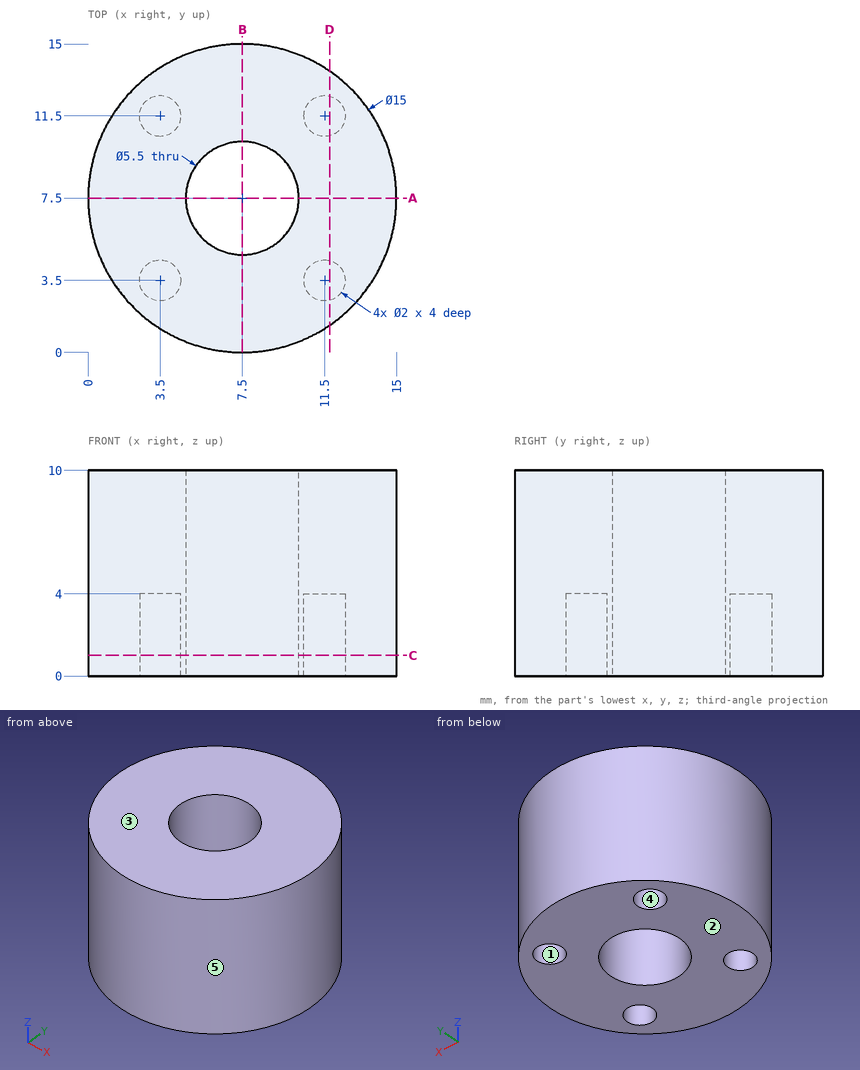
Study the drawing (mm; zero at the part's minimum x, y, z) and answer. A direction names the side the tool comes from. Round coordinates to 2 decimals unless told otherwise and drop trailing zeros. Write each loop counter-clockwise with the first axis right and the second up, starting at its lowest first coordinate (ties: lowest second). Pieces come first, ordered by that corner, then holes. Notation, with made-up numbers: (-2, 77) - (20, 77) arc R24 cw to (20, 113) - close; hole circle Ø9 at (-8.5, 39). An arc over 180 degrees is marked (long way). Use a Markdown table: item, result. Add a question column.
1. Flat-ended cylindrical pins translate along their axes: P1, Ø5, axis at x = 13, z = 4, coming from the +Y side; P2, Ø2, axis at x = 11.5, y = 11, coming from the -Z side; P3, Ø1.5, axis at x = 6, z = 3.5, coming from the -Y side; P4, Ø1.5, axis at y = 11, z = 2.5, coming from the -X side. Find the tip coordinate at first contact, or state that the pin passes through.
2. Consider line 1 (X direction, y = 4, z = 0.5); line 2 (Y direction, x = 3.5, z = 2.75); line 3 (Y direction, x = 7.5, z = 2.5). Determine where each line is inside the solid, lowest interval first.
3. The part is cut by section C-C (z = 1). Write down the section's boundary in (x, y).
4. For a pull along X with two mould halves and no side action, classify the marked faces 3, 4 and 5 as +X half, -X half, draft (parallel to the pull), parting line (faces both ways), or undercut.
5. A tool of negligible diameter and unlimited length cuts with its end or side. For the marked faces 1 and 2, from which of +Z, -Z, +X, -X, +Y, -Y can it reach the whole face along a straight path? Write none if from no direction.
6. The part is cut by section D-D (x = 11.75). Write down the section's boundary in (y, z), and give its area (3 significant figures).
7. The part is cut by section A-A (y = 7.5). Write down the section's boundary in (x, z).
Reported:
| question | item | result |
|---|---|---|
| 1 | P1 | y = 14.37 |
| 1 | P2 | z = 0 |
| 1 | P3 | y = 0.04 |
| 1 | P4 | x = 0.52 |
| 2 | line 1 | 0.87 to 2.63, 4.37 to 10.63, 12.37 to 14.13 |
| 2 | line 2 | 1.16 to 2.5, 4.5 to 10.5, 12.5 to 13.84 |
| 2 | line 3 | 0 to 4.75, 10.25 to 15 |
| 3 | outline | circle Ø15 at (7.5, 7.5); hole circle Ø2 at (3.5, 3.5); hole circle Ø2 at (3.5, 11.5); hole circle Ø5.5 at (7.5, 7.5); hole circle Ø2 at (11.5, 3.5); hole circle Ø2 at (11.5, 11.5) |
| 4 | face 3 | draft |
| 4 | face 4 | undercut |
| 4 | face 5 | parting line |
| 5 | face 1 | -Z |
| 5 | face 2 | -Z, +X, -X, +Y, -Y |
| 6 | outline | (1.32, 0) - (2.53, 0) - (2.53, 4) - (4.47, 4) - (4.47, 0) - (10.53, 0) - (10.53, 4) - (12.47, 4) - (12.47, 0) - (13.68, 0) - (13.68, 10) - (1.32, 10) - close |
| 6 | area | 108 mm^2 |
| 7 | outline | (0, 0) - (4.75, 0) - (4.75, 10) - (0, 10) - close; (10.25, 0) - (15, 0) - (15, 10) - (10.25, 10) - close |
